```python
from build123d import *

# Parameters (mm, degrees)
SKETCH1_R               = 7.1
SKETCH1_R_2             = 3.1
BOSS_EXTRUDE1_DEPTH     = 20
SKETCH3_R               = 1.15
CUT_EXTRUDE1_DEPTH      = 8.1
CUT_EXTRUDE1_DEPTH_BACK = 8.1
CUT_EXTRUDE2_START      = -4
SKETCH5_R               = 1.8
CUT_EXTRUDE2_DEPTH      = 5
SKETCH2_R               = 7.1
BOSS_EXTRUDE2_DEPTH     = 5
CHAMFER1_SIZE           = 2


with BuildPart() as part:
    # Sketch1 → Boss-Extrude1 (new body)
    with BuildSketch(Plane(origin=(0, 0, 0), x_dir=(1, 0, 0), z_dir=(0, 1, 0))):
        Circle(SKETCH1_R)
        Circle(SKETCH1_R_2, mode=Mode.SUBTRACT)
    extrude(amount=BOSS_EXTRUDE1_DEPTH)

    # Sketch3 → Cut-Extrude1 (cut, two sides)
    with BuildSketch(Plane.XY) as cut_extrude1_sk:
        with Locations((0, 5.3)):
            Circle(SKETCH3_R)
    extrude(amount=CUT_EXTRUDE1_DEPTH, mode=Mode.SUBTRACT)
    extrude(cut_extrude1_sk.sketch, amount=-CUT_EXTRUDE1_DEPTH_BACK, mode=Mode.SUBTRACT)

    # Sketch5 → Cut-Extrude2 (cut)
    with BuildSketch(Plane.XY.offset(CUT_EXTRUDE2_START)):
        with Locations((0, 5.3)):
            Circle(SKETCH5_R)
    extrude(amount=-CUT_EXTRUDE2_DEPTH, mode=Mode.SUBTRACT)

    # Sketch2 → Boss-Extrude2 (add)
    with BuildSketch(Plane.XZ):
        Circle(SKETCH2_R)
    extrude(amount=BOSS_EXTRUDE2_DEPTH)

    # Chamfer1
    chamfer1_edges = [part.edges().sort_by_distance(p)[0] for p in [
        (-7.1, -5, 0),
        (-7.1, 20, 0),
    ]]
    chamfer(chamfer1_edges, length=CHAMFER1_SIZE)


solid = part.part
```
Work out the finished part from the listing and answer in its coordinate system (mm). Give positions to 0.01 mm unless a question says otherwise; leave off trailing zeros. Loops run counter-clockwise (first coordinate to the right, second up) from the corner with the lowest first, then second, coordinate; pieces in that order, holes last. Notation, with made-up numbers: (16, 36.25) -> (66, 36.25) arc R28 ccw to (66, 61.25) -> close; hole circle Ø8 at (85, 56). An arc over 180 degrees is marked (long way). Use CSV: the item, a comma, the result in double quotes.
1. Straight lines are drawn through the part: line 1 (X direction, y = 9.75, z = 0); line 2 (Y direction, x = 0, z = 0.5); line 3 (X direction, y = 5.3, z = -6.5). For each, find the intervals that lie inside material, in ascending order.
Found:
line 1,"-7.1 to -3.1, 3.1 to 7.1"
line 2,"-5 to 0"
line 3,"-2.86 to -1.8, 1.8 to 2.86"
2. The mould has two halves that part along Z. Classify faces 1 (the cylindrical face through (-1.8, 5.38, -5.53)), 2 (the flat face through (0, 4, -4)), 3 (the cylindrical face through (2.957, 9.86, -0.931)), 4 (the flat face through (0, 0, 0)): +Z half, -Z half, draft (parallel to the pull), parting line (faces both ways), or undercut.
Found:
face 1,"draft"
face 2,"-Z half"
face 3,"undercut"
face 4,"undercut"
3. The part is cut by section D-D (y = 11). Write down the section's boundary in (x, z).
Found:
outline,"circle Ø14.2 at (0, 0); hole circle Ø6.2 at (0, 0)"
4. The part is cut by section C-C (z = 0). Write down the section's boundary in (x, y).
Found:
outline,"(-7.1, -3) -> (-5.1, -5) -> (5.1, -5) -> (7.1, -3) -> (7.1, 18) -> (5.1, 20) -> (3.1, 20) -> (3.1, 0) -> (-3.1, 0) -> (-3.1, 20) -> (-5.1, 20) -> (-7.1, 18) -> close"
5. The part is cut by section A-A (x = 0). Write down the section's boundary in (y, z), then the cut area to 3 significant figures.
Found:
outline,"(-5, -5.1) -> (-3, -7.1) -> (3.5, -7.1) -> (3.5, -4) -> (4.15, -4) -> (4.15, -3.1) -> (0, -3.1) -> (0, 3.1) -> (4.15, 3.1) -> (4.15, 7.1) -> (-3, 7.1) -> (-5, 5.1) -> close; (6.45, -4) -> (7.1, -4) -> (7.1, -7.1) -> (18, -7.1) -> (20, -5.1) -> (20, -3.1) -> (6.45, -3.1) -> close; (6.45, 3.1) -> (20, 3.1) -> (20, 5.1) -> (18, 7.1) -> (6.45, 7.1) -> close"
area,"201 mm^2"
6. The part is cut by section B-B (y = 5.3). Write down the section's boundary in (x, z).
Found:
outline,"(-1.8, -6.87) -> (-1.8, -4) -> (-1.15, -4) -> (-1.15, -2.88) arc R3.1 cw to (-1.15, 2.88) -> (-1.15, 7.01) arc R7.1 ccw to start; (1.15, -4) -> (1.8, -4) -> (1.8, -6.87) arc R7.1 ccw to (1.15, 7.01) -> (1.15, 2.88) arc R3.1 cw to (1.15, -2.88) -> close"
7. Flat-ended cylindrical pins translate along their axes: pin 1 Ø6 at (x, y) = (-5.5, 4.5) entering from +Z; pin 2 Ø1.5 at (x, y) = (1.5, 1) entering from -Z; pin 3 Ø1 at (x, y) = (1, 14.5) entering from +Z. Find the tip coordinate at first contact, or state that the pin passes through.
Found:
pin 1,"z = 6.65"
pin 2,"z = -7.06"
pin 3,"z = 7.08"
